Build history of the part. All positions in model axes, mm. A direction names the side the tool comes from. Coordinates: 2 decimals unless noted, no trailing zeros. Write each loop counter-clockwise with the first axis right and the second up, starting at its lowest first coordinate (ties: lowest second). Pieces come first, ordered by that corner, then holes.
from build123d import *

# Parameters (mm, degrees)
CHAMFER_1_SIZE           = 2
SKETCH_2_R               = 10
CUT_EXTRUDE_1_DEPTH      = 10
PATTERN_CIRCULAR_1_COUNT = 3
CUT_EXTRUDE_2_DEPTH      = 214.395173329
CUT_EXTRUDE_2_DEPTH_BACK = 214.395173329
SKETCH_3_W               = 40
SKETCH_3_H               = 24.854018102


with BuildPart() as part:
    # Эскиз1 → Повернуть1 (revolve)
    with BuildSketch(Plane.XY, mode=Mode.PRIVATE) as revolve_1_sk:
        Polygon((77.5, 30), (77.5, 0), (117.5, 0), (132.5, -15), (147.5, -15), (147.5, -7.5), (110, 30), align=None)
    revolve(revolve_1_sk.sketch.rotate(Axis((0, 107.750556793, 0), (0, -1, 0)), 90), axis=Axis((0, 107.750556793, 0), (0, -1, 0)))

    # Фаска1
    chamfer_1_edges = [part.edges().sort_by_distance(p)[0] for p in [
        (0, 0, -77.5),
        (0, 30, -77.5),
    ]]
    chamfer(chamfer_1_edges, length=CHAMFER_1_SIZE)

    # Эскиз2 → Вырез-Вытянуть1 (cut)
    with BuildSketch(Plane(origin=(0, 30, 0), x_dir=(1, 0, 0), z_dir=(0, 1, 0))):
        with Locations(Location((0, 95, 0), (0, 0, 270))):
            Circle(SKETCH_2_R)
    cut_extrude_1 = extrude(amount=-CUT_EXTRUDE_1_DEPTH, mode=Mode.SUBTRACT)

    # Круговой массив1: Вырез-Вытянуть1 ×3 about axis
    pattern_circular_1_axis = Axis((0, 0, 0), (0, 1, 0))
    for i in range(1, PATTERN_CIRCULAR_1_COUNT):
        add(cut_extrude_1.rotate(pattern_circular_1_axis, i * 360 / PATTERN_CIRCULAR_1_COUNT), mode=Mode.SUBTRACT)

    # Эскиз3 → Вырез-Вытянуть2 (cut, two sides: drawn at the far end of the back side and taken through both)
    with BuildSketch(Plane(origin=(0, 30, 0), x_dir=(1, 0, 0), z_dir=(0, 1, 0)).offset(-CUT_EXTRUDE_2_DEPTH_BACK)):
        with Locations((0, -74.472990949)):
            Rectangle(SKETCH_3_W, SKETCH_3_H)
    extrude(amount=CUT_EXTRUDE_2_DEPTH + CUT_EXTRUDE_2_DEPTH_BACK, mode=Mode.SUBTRACT)


solid = part.part
(1) Slice it at B-B, the plane x = 0. List the corners of the cut face in (y, z).
(2) Probe L1, parallel to X at y = 26, z = 47; L2, parallel to Y at x = 25, z = -90; L3, parallel to X at y = 19.5, z = 34.5. List the from-to ranges inside material, lowest first.
(3) 3-axis set-ups, long thin cutter, end or side, ignore diameter. For faces 4 (the flat face through (0, 15, 86.9)), 5 (the cylindrical face through (-72.358, 25.07, 46.198)), 6 (the flat face through (24, 0, -77)): which of +Z, -Z, +X, -X, +Y, -Y reach the whole face in a straight line?
(4) Slice it at C-C, the plane y = 8.5. List the corners of the cut face in (x, z).
(5) Flat gauge pins, fed straight in: P1, Ø2, axis at y = -5, z = 4, coming from the +X side; P2, Ø6, axis at x = -83.5, z = 43.5, coming from the +Y side; P3, Ø5, axis at y = 10.5, z = 56, coming from the +X side. Where does each tip first touch, or does it go through?
(6) Two-plate mould, pull along Z, no slides. Class faces 1 (the flat face through (-74, 30, 32)), 2 (the conical face through (-110.87, 28.18, -14.56)), 3 (the flat face through (82, 20, 48)): pulls with the +Z half, pulls with the -Z half, needs draft (parallel to the pull), parting line crosses it, or undercut.
(7) Slice it at A-A, the plane z = 0. List the corners of the cut face in (x, y).
Results:
1. outline: (-15, -147.5) - (-7.5, -147.5) - (30, -110) - (30, -105) - (20, -105) - (20, -85) - (30, -85) - (30, -79.5) - (28, -77.5) - (2, -77.5) - (0, -79.5) - (0, -117.5) - (-15, -132.5) - close; (-15, 132.5) - (0, 117.5) - (0, 86.9) - (30, 86.9) - (30, 110) - (-7.5, 147.5) - (-15, 147.5) - close
2. L1: x = -103.86 to -92.26, -72.28 to -61.62, 61.62 to 72.28, 92.26 to 103.86
2. L2: y = 0 to 30
2. L3: x = -115.46 to -69.4, 69.4 to 115.46
3. face 4: +Y, -Y
3. face 5: +Y
3. face 6: -Y
4. outline: circle Ø263 at (0, 0); hole (-20, 74.87) arc R77.5 ccw (long way) to (20, 74.87) - (20, 86.9) - (-20, 86.9) - close
5. P1: stops at x = 145.95
5. P2: stops at y = 20
5. P3: stops at x = 119.77
6. face 1: needs draft
6. face 2: parting line crosses it
6. face 3: undercut
7. outline: (-147.5, -15) - (-132.5, -15) - (-117.5, 0) - (-79.5, 0) - (-77.5, 2) - (-77.5, 28) - (-79.5, 30) - (-110, 30) - (-147.5, -7.5) - close; (77.5, 2) - (79.5, 0) - (117.5, 0) - (132.5, -15) - (147.5, -15) - (147.5, -7.5) - (110, 30) - (79.5, 30) - (77.5, 28) - close
